```python
from build123d import *

# Parameters (mm, degrees)
F0_W     = 96
F0_H     = 26
F1_DEPTH = 5
F3_D     = 4
F5_D     = 3


with BuildPart() as f1:
    # F0 (on Top) → F1 (new body)
    with BuildSketch(Plane.XY):
        Rectangle(F0_W, F0_H)
    extrude(amount=F1_DEPTH)

    # F3 (through all)
    with Locations(Plane.XY.offset(5)):
        with Locations((-43, 9), (-19, 9), (19, 9), (43, 9), (43, -9), (19, -9), (-19, -9), (-43, -9)):
            Hole(F3_D / 2)

    # F5 (through all)
    with Locations(Plane.XY.offset(5)):
        with Locations((-31, 9), (0, -9), (31, 9)):
            Hole(F5_D / 2)


solid = f1.part
```
For this review, take the finished solid that the model builds, in its own axes (mm). Coordinates: 2 decimals unless noted, no trailing zeros. Order: outer loops, then holes, each group sorted by start corner. A loop starts at its lowest first (then second) coordinate and runs counter-clockwise, first axis right, second up. Notation, with made-up numbers: (8.25, 10) -> (54.25, 10) arc R17 ccw to (54.25, 38) -> close; hole circle Ø8 at (-37.5, -30.75). An arc over 180 degrees is marked (long way). Answer as CSV lines item,"result".
Q1. We need section A-A (x = 31). State the section outline as (y, z) points.
Model answer:
outline,"(-13, 0) -> (7.5, 0) -> (7.5, 5) -> (-13, 5) -> close; (10.5, 0) -> (13, 0) -> (13, 5) -> (10.5, 5) -> close"
Q2. We need section B-B (z = 1.7). Count the separate pieces of the cut face and the enclosed holes in it, plus the area to 3 significant figures.
Model answer:
separate pieces,"1"
enclosed holes,"11"
area,"2,370 mm2"
Q3. Draft analysis for pull direction X (two halves, no side actions). For faces 1 (the face through (44.474, 10.352, 2.465)), 2 (the face through (48, 0, 2)), 3 (the face through (-1, 0, 0)), state which applies: released by +X, released by -X, zero draft, split by the parting line, or undercut.
Model answer:
face 1,"undercut"
face 2,"released by +X"
face 3,"zero draft"
Q4. We need section D-D (y = -9). State the section outline as (x, z) points.
Model answer:
outline,"(-48, 0) -> (-45, 0) -> (-45, 5) -> (-48, 5) -> close; (-41, 0) -> (-21, 0) -> (-21, 5) -> (-41, 5) -> close; (-17, 0) -> (-1.5, 0) -> (-1.5, 5) -> (-17, 5) -> close; (1.5, 0) -> (17, 0) -> (17, 5) -> (1.5, 5) -> close; (21, 0) -> (41, 0) -> (41, 5) -> (21, 5) -> close; (45, 0) -> (48, 0) -> (48, 5) -> (45, 5) -> close"
Q5. We need section C-C (x = 43). State the section outline as (y, z) points.
Model answer:
outline,"(-13, 0) -> (-11, 0) -> (-11, 5) -> (-13, 5) -> close; (-7, 0) -> (7, 0) -> (7, 5) -> (-7, 5) -> close; (11, 0) -> (13, 0) -> (13, 5) -> (11, 5) -> close"
Q6. Wall thickness on line 1 along Y through (x, z) = (19, 3); line 2 along X through (y, z) = (-7.25, 3.5); line 3 along Y through (x, z) = (-31, 3): over which ranges is each line inside the solid? List them lowest first. Write a range as [from, to].
Model answer:
line 1,"y = [-13, -11], [-7, 7], [11, 13]"
line 2,"x = [-48, -43.97], [-42.03, -19.97], [-18.03, 18.03], [19.97, 42.03], [43.97, 48]"
line 3,"y = [-13, 7.5], [10.5, 13]"
